from build123d import *

# Parameters (mm, degrees)
F0_W     = 32
F0_H     = 9
F1_DEPTH = 280
F3_DEPTH = 280


with BuildPart() as f1:
    # F0 (on Front) → F1 (new body)
    with BuildSketch(Plane.XZ):
        Polygon((-41.5, -22.5), (-39.5, -22.5), (-39.5, -12.5), (-35.5, -12.5), (-35.5, -22.5), (-33.5, -22.5), (-33.5, -12.5), (-31.5, -12.5), (-31.5, -18.5), (-29.5, -18.5), (-29.5, -12.5), (-9.75, -12.5), (-9.75, -14.5), (-7.75, -14.5), (-7.75, -12.5), (0, -12.5), (0, 18.5), (-0.75, 18.5), (-1.000473, 3.5), (-5.75, 3.5), (-5.999527, 18.5), (-7.499527, 18.5), (-7.75, 3.5), (-12.5, 3.5), (-12.749527, 18.5), (-14.249527, 18.5), (-14.5, 3.5), (-19.25, 3.5), (-19.499527, 18.5), (-20.999527, 18.5), (-21.25, 3.5), (-26, 3.5), (-26.249527, 18.5), (-27.749527, 18.5), (-28, 3.5), (-32.75, 3.5), (-32.999527, 18.5), (-34.499527, 18.5), (-34.75, 3.5), (-39.5, 3.5), (-39.749527, 18.5), (-41.249527, 18.5), (-41.5, 3.5), align=None)
        with Locations((-19.5, -4.5)):
            Rectangle(F0_W, F0_H, mode=Mode.SUBTRACT)
    extrude(amount=F1_DEPTH)

    # F2 (on Front) → F3 (join)
    with BuildSketch(Plane.XZ):
        Polygon((-46.5, -12.194781), (-41.5, -12.194781), (-41.5, -10.194781), (-46.37868, -10.194781), (-52.43934, -4.134121), (-53.5, -5.194781), align=None)
        Polygon((-53.5, 1.555219), (-46.5, -5.444781), (-41.5, -5.444781), (-41.5, -3.444781), (-46.37868, -3.444781), (-52.43934, 2.615879), align=None)
        Polygon((-53.5, 8.305219), (-46.5, 1.305219), (-41.5, 1.305219), (-41.5, 3.305219), (-46.37868, 3.305219), (-52.43934, 9.365879), align=None)
    extrude(amount=F3_DEPTH)

    # F4: F1 across face


with BuildPart() as f1_1:
    add(f1.part)
    add(f1.part.mirror(Plane(origin=(0, -140, 3), x_dir=(0, 1, 0), z_dir=(1, 0, 0))))


solid = f1_1.part
Verification items for the finished model (mm, model axes). A direction names the side the tool comes from. Coordinates: 2 decimals unless noted, no trailing zeros. Use CSV: the item, a comma, the result in double quotes.
Q1. Go/stop test with flat-tipped pins: P1, Ø5, axis at y = -47, z = 12, coming from the -X side; P2, Ø8, axis at y = -141, z = -16, coming from the -X side; P3, Ø1.5, axis at x = -43.5, y = -77, coming from the +Z side. Record where each tip stops, or that it passes through.
Computed values:
P1,"x = -41.4"
P2,"x = -46.69"
P3,"z = 3.31"
Q2. Mould release check, pull along X, two halves, no side actions. Record for faces 4 (the flat face through (30, -138, 3.5)), 5 (the flat face through (-41.5, -138, -17)), 6 (the flat face through (41.5, -138, -17)): pulls with the +X half, pulls with the -X half, needs draft (parallel to the pull), parting line crosses it, or undercut.
Computed values:
face 4,"undercut"
face 5,"pulls with the -X half"
face 6,"pulls with the +X half"
Q3. Thickness scan on line 1 along Z through (x, y) = (43.5, -45.5); line 2 along Z through (x, y) = (14, -62.5); line 3 along X through (y, z) = (-42, 2.5). Record the ranges inside material, lowest first. Write a range as [from, to].
Computed values:
line 1,"[-12.19, -10.19], [-5.44, -3.44], [1.31, 3.31]"
line 2,"[-12.5, -9], [0, 18.5]"
line 3,"[-52.56, -52.32], [-47.69, 47.69], [52.32, 52.56]"
Q4. Set-up check for faces 1 (the flat face through (-17, -138, 3.5)), 2 (the flat face through (-44, -138, -3.445)), 3 (the flat face through (35.5, -138, -17)): record each of +Z, -Z, +X, -X, +Y, -Y from which the full face is reachable in a straight line by a thin tool's end or side.
Computed values:
face 1,"+Z, +Y, -Y"
face 2,"+Y, -Y"
face 3,"-Z, +Y, -Y"
Q5. Section check A-A, the plane y = -147. State how many separate pieces and enclosed holes the cut face has, and give its area (3 significant figures).
Computed values:
separate pieces,"1"
enclosed holes,"2"
area,"1,350 mm²"
